Geometry: final body of the model. Coordinates: model frame, mm. A direction names the side the tool comes from. Coordinates: 2 decimals unless noted, no trailing zeros. Order: outer loops, then holes, each group sorted by start corner. A loop starts at its lowest first (then second) coordinate and runs counter-clockwise, first axis right, second up. Notation, with made-up numbers: (52, 25.25) - (84, 25.25) arc R22 ccw to (84, 54.25) - close; hole circle Ø4 at (73, -15). An arc over 180 degrees is marked (long way). Use a Markdown table: item, result. Add a question column.
Autodesk Inventor part; units mm, degrees
ref_plane "YZ Plane" through (0, 0, 0) normal (1, 0, 0) x (0, 1, 0)
ref_plane "XZ Plane" through (0, 0, 0) normal (0, 1, 0) x (-1, 0, 0)
ref_plane "XY Plane" through (0, 0, 0) normal (0, 0, 1) x (1, 0, 0)
sketch "Sketch1" plane through (0, 0, 0) normal (1, 0, 0) x (0, 1, 0)
  line L0 (0, 0) -> (0, -35.075)
  line L1 (0, -35.075) -> (2, -35.075)
  line L2 (19.925, 20.075) -> (40.075, 20.075)
  line L3 (40.075, 20.075) -> (40.075, -20.075)
  line L4 (40.075, -20.075) -> (19.925, -20.075)
  line L5 (19.925, -20.075) -> (19.925, 20.075)
  line L6 (19.925, 20.075) -> (40.075, -20.075) construction
  line L7 (40.075, 20.075) -> (19.925, -20.075) construction
  line L8 (16.925, 23.075) -> (43.075, 23.075)
  line L9 (43.075, 23.075) -> (43.075, -23.075)
  line L10 (43.075, -23.075) -> (16.925, -23.075)
  line L11 (16.925, -23.075) -> (16.925, 23.075)
  line L12 (16.925, 23.075) -> (43.075, -23.075) construction
  line L13 (43.075, 23.075) -> (16.925, -23.075) construction
  line L14 (0, 0) -> (0, 35.075)
  line L15 (0, 35.075) -> (2, 35.075)
  arc A0 (2, 35.075) -> (43.075, 23.075) centre (41.5508, 94.1558) ccw
  arc A1 (43.075, -23.075) -> (2, -35.075) centre (42.3004, -96.7217) ccw
  line L16 (-8.615, 0) -> (51.69, 0)
  point P0 (20, 0)
  point P1 (40.1, 0)
  point P2 (30, 0)
  point P3 (30, 23.075)
  point P4 (30.025, -23.075)
  point P5 (30, 0)
  dimension "d0" = 35.075
  dimension "d1" = 2
  dimension "d2" = 20
  dimension "d4" = 20.15
  dimension "d5" = 40.15
  dimension "d6" = 46.15
  dimension "d7" = 26.15
  dimension "d8" = 35.075
extrude "Extrusion1" add sketch "Sketch1" along normal blind 20 contours L10 L11 L16 L5 L4 L3 L9 | L16 L11 L10 A1 L1 L0 | L14 L15 A0 L8 L11 L16 | L11 L8 A0 L9 L16 L3 L2 L5 | L8 A0
sketch "Sketch2" plane through (0, 43.075, 23.075) normal (0, 1, 0) x (1, 0, 0)
  line L0 (0, 46.15) -> (0, 0)
  line L1 (0, 0) -> (20, 0)
  line L2 (20, 46.15) -> (20, 0)
  line L3 (0, 46.15) -> (20, 46.15)
  line L4 (0, 3) -> (20, 3)
  line L5 (0, 3) -> (20, 3)
  point P0 (0, 23.075)
  point P1 (10, 13.05)
  point P2 (10, 33.05)
  dimension "d33" = 20
  dimension "d34" = 10.05
hole "Hole1" at (10, 43.075, 10.025) at (10, 43.075, -9.975) direction (0, -1, 0) diameter 4 end up to surface
ref_plane "Work Plane1" through (0, 11, -35.075) normal (0, -1, 0) x (1, 0, 0)
sketch "Sketch3" plane through (0, 11, -35.075) normal (0, -1, 0) x (1, 0, 0)
  circle A0 centre (10, 45.1) radius 2
  line L0 (0, 12) -> (0, 58.15)
  line L1 (0, 58.15) -> (20, 58.15)
  line L2 (20, 12) -> (20, 58.15)
  line L3 (0, 12) -> (20, 12)
  line L4 (0, 55.15) -> (0, 15)
  line L5 (0, 55.15) -> (20, 55.15)
  line L6 (20, 15) -> (20, 55.15)
  line L7 (0, 15) -> (20, 15)
  circle A1 centre (10, 62.15) radius 4
  circle A2 centre (10, 8) radius 4
  point P0 (0, 35.075)
  dimension "d19" = 4
  dimension "d20" = 4
  dimension "d30" = 8
  dimension "d31" = 8
extrude "Extrusion2" cut sketch "Sketch3" against normal blind 20 contours A1 | A2
hole "Hole2" at (10, 11, 27.075) at (10, 11, -27.075) direction (0, -1, 0) diameter 4.5 end through all
chamfer "Chamfer1" distance 1 angle 45 4 edges at (20, 40.075, 0) (20, 30, 20.075) (20, 19.925, 0) (20, 30, -20.075)
sketch "Sketch4" plane through (20, 0, 0) normal (1, 0, 0) x (0, 0, -1)
  line L0 (0, -8.615) -> (0, 51.69)
  line L1 (-35.075, 0) -> (35.075, 0)
  line L2 (0, 0) -> (2, 2)
  line L3 (2, 2) -> (-2, 2)
  line L4 (-2, 2) -> (0, 0)
extrude "Extrusion3" add sketch "Sketch4" along normal blind 0.4
sketch "Sketch5" plane through (20, 0, 0) normal (1, 0, 0) x (0, 0, -1)
  line L0 (0, 0) -> (35.075, 0)
  line L1 (35.075, 0) -> (35.075, 2)
  point P0 (27.075, 5)
  dimension "d42" = 5
  dimension "d43" = 8
hole "Hole3" at (20, 5, -27.075) direction (-1, 0, 0) diameter 3.5 depth 5
equation "\"d8\" = d0"
equation "\"d31\" = d30"
properties part number "espaceur_20mm_v3"
1) Draft query along X for faces 1 (the face through (8.1, 5.42, 28.28)), 2 (the face through (20.4, 1, 0)), 3 (the face through (0, 16, 0)), 4 (the face through (10, 1, -35.075)). Return one class per face: pulls with the +X half, pulls with the -X half, needs draft (parallel to the pull), parting line crosses it, or undercut.
2) Pin query (flat end, axial travel): pin 1 (3 mm diameter, centred on x = 3.5, y = 32, fed in from +Z); pin 2 (1.5 mm diameter, centred on x = 8.5, y = 41, fed in from +Z) (3 decimals); pin 3 (4 mm diameter, centred on y = 5, z = -27.5, fed in from +X). Return the tip coordinate at first contact, or that it passes through.
3) Section D-D (y = 21.5). Return loops of the section in (x, z) (3 decimals), then the cut area to 3 significant figures.
4) Ray query, line 1 along Z through (x, y) = (10, 41.15) (3 decimals); line 2 along Y through (x, z) = (13.5, -12.5) (3 decimals); line 3 along Z through (x, y) = (15.75, 36) (3 decimals). Return the intervals inside material, ascending.
5) Section A-A (x = 17.75). Return loops of the section in (y, z) (3 decimals).
6) Section C-C (y = 7.5). Return loops of the section in (x, z) (3 decimals).
7) Section B-B (x = 2). Return loops of the section in (y, z) (3 decimals).
8) Set-up query: faces 5 (the face through (17.465, 6.065, -25.686)), 6 (the face through (9.867, 18.638, 23.077)), 7 (the face through (20.2, 1, 1)), 8 (the face through (10, 42, 23.075)). Return all of +Z, -Z, +X, -X, +Y, -Y with unobstructed straight access to the full face (end or side cutting, diameter ignored); none if empty.
Values follow:
| question | item | result |
|---|---|---|
| 1 | face 1 | undercut |
| 1 | face 2 | pulls with the +X half |
| 1 | face 3 | pulls with the -X half |
| 1 | face 4 | needs draft |
| 2 | pin 1 | stops at z = 23.92 |
| 2 | pin 2 | stops at z = 23.075 |
| 2 | pin 3 | stops at x = 20 |
| 3 | outline | (0, -26.069) - (6.129, -26.069) arc R4 cw to (13.871, -26.069) - (20, -26.069) - (20, -21.075) - (19, -20.075) - (0, -20.075) - close; (0, 20.075) - (19, 20.075) - (20, 21.075) - (20, 25.945) - (13.837, 25.945) arc R4 cw to (6.163, 25.945) - (0, 25.945) - close |
| 3 | area | 203 mm² |
| 4 | line 1 | z = -23.08 to -11.975, -7.975 to 8.025, 12.025 to 23.075 |
| 4 | line 2 | y = 0 to 19.925, 40.075 to 43.075 |
| 4 | line 3 | z = -23.341 to -20.075, 20.075 to 23.276 |
| 5 | outline | (0, -35.075) - (2, -35.075) arc R73.651 cw to (43.075, -23.075) - (43.075, 23.075) - (40.026, 23.075) arc R71.097 cw to (2, 35.075) - (0, 35.075) - close; hole circle Ø3.5 at (5, -27.075); hole (19.925, -20.075) - (40.075, -20.075) - (40.075, 20.075) - (19.925, 20.075) - close |
| 6 | outline | (0, -31.811) - (20, -31.811) - (20, 31.743) - (0, 31.743) - close; hole circle Ø4.5 at (10, -27.075); hole circle Ø4.5 at (10, 27.075) |
| 7 | outline | (0, -35.075) - (2, -35.075) arc R73.651 cw to (43.075, -23.075) - (43.075, 23.075) - (40.026, 23.075) arc R71.097 cw to (2, 35.075) - (0, 35.075) - close; hole (19.925, -20.075) - (40.075, -20.075) - (40.075, 20.075) - (19.925, 20.075) - close |
| 8 | face 5 | +X |
| 8 | face 6 | none |
| 8 | face 7 | +Z, +X, -Y |
| 8 | face 8 | +Z, +X, -X, +Y |
